from build123d import *

# Parameters (mm, degrees)
SKETCH1_R           = 3.25
BOSS_EXTRUDE1_DEPTH = 8
BOSS_EXTRUDE2_DEPTH = 12.5
BOSS_EXTRUDE3_START = -12.5
BOSS_EXTRUDE3_DEPTH = 8
SKETCH2_R           = 7.5
BOSS_EXTRUDE4_DEPTH = 10
FILLET2_R           = 2
FILLET3_R           = 5


with BuildPart() as part:
    # Sketch1 → Boss-Extrude1 (new body)
    with BuildSketch(Plane(origin=(0, 0, 0), x_dir=(1, 0, 0), z_dir=(0, 1, 0))):
        with BuildLine():
            Line((-20, 10), (-20, -10))
            Line((-20, -10), (-11.180339887, -10))
            ThreePointArc((-11.180339887, -10), (0, -15), (11.180339887, -10))
            Line((11.180339887, -10), (20, -10))
            Line((20, -10), (20, 10))
            Line((20, 10), (11.180339887, 10))
            ThreePointArc((11.180339887, 10), (0, 15), (-11.180339887, 10))
            Line((-11.180339887, 10), (-20, 10))
        make_face()
        with Locations(Location((0, 0, 0), (0, 0, 270))):
            Circle(SKETCH1_R, mode=Mode.SUBTRACT)
    extrude(amount=BOSS_EXTRUDE1_DEPTH)

    # Sketch1<3> → Boss-Extrude2 (add)
    with BuildSketch(Plane(origin=(0, 0, 0), x_dir=(1, 0, 0), z_dir=(0, 1, 0))):
        Polygon((-15, 10), (-20, 10), (-20, -10), (-15, -10), (-15, 0), align=None)
        Polygon((20, 10), (15, 10), (15, 0), (15, -10), (20, -10), align=None)
    extrude(amount=-BOSS_EXTRUDE2_DEPTH)

    # Sketch1<4> → Boss-Extrude3 (add)
    with BuildSketch(Plane(origin=(0, 0, 0), x_dir=(1, 0, 0), z_dir=(0, 1, 0)).offset(BOSS_EXTRUDE3_START)):
        with BuildLine():
            Line((-20, 10), (-20, -10))
            Line((-20, -10), (-11.180339887, -10))
            ThreePointArc((-11.180339887, -10), (0, -15), (11.180339887, -10))
            Line((11.180339887, -10), (20, -10))
            Line((20, -10), (20, 10))
            Line((20, 10), (11.180339887, 10))
            ThreePointArc((11.180339887, 10), (0, 15), (-11.180339887, 10))
            Line((-11.180339887, 10), (-20, 10))
        make_face()
    extrude(amount=-BOSS_EXTRUDE3_DEPTH)

    # Sketch2 → Boss-Extrude4 (add)
    with BuildSketch(Plane.XZ.offset(20.5)):
        with Locations(Location((0, 0, 0), (0, 0, 270))):
            Circle(SKETCH2_R)
    extrude(amount=BOSS_EXTRUDE4_DEPTH)

    # Sketch3 → Revolve1 (revolve)
    with BuildSketch(Plane.XY):
        with BuildLine():
            ThreePointArc((0, -28.863068172), (-3.8382791, -29.277061987), (-7.5, -30.5))
            Line((-7.5, -30.5), (0, -30.5))
            Line((0, -30.5), (0, -28.863068172))
        make_face()
        with BuildLine():
            Line((0, -30.5), (-7.5, -30.5))
            ThreePointArc((-7.5, -30.5), (-17.586006185, -50.701347272), (0, -64.863068172))
            Line((0, -64.863068172), (0, -30.5))
        make_face()
    revolve(axis=Axis((0, -64.863068172, 0), (0, 1, 0)))

    # Fillet2
    fillet2_edges = [part.edges().sort_by_distance(p)[0] for p in [
        (-20, -6.25, -10),
        (-20, -6.25, 10),
        (15.590169944, -20.5, 10),
        (0, -20.5, -15),
        (0, -20.5, 15),
        (-15.590169944, -20.5, -10),
        (15.590169944, -20.5, -10),
        (20, -20.5, 0),
        (-20, -20.5, 0),
        (20, -6.25, -10),
        (-15.590169944, -20.5, 10),
        (20, -6.25, 10),
    ]]
    fillet(fillet2_edges, radius=FILLET2_R)

    # Fillet3
    fillet3_edges = [part.edges().sort_by_distance(p)[0] for p in [
        (0, -20.5, 7.5),
        (-5.303300859, -30.5, -5.303300859),
    ]]
    fillet(fillet3_edges, radius=FILLET3_R)


solid = part.part
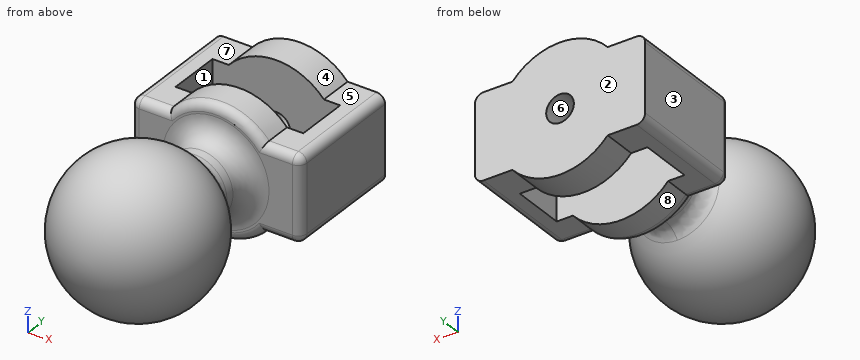
Design review of the part built by this model. Coordinates are the model's own, in mm. Face numbers are marked on the shaded views. A direction names the side the tool comes from. Give positions to 0.01 mm unless a question says otherwise; leave off trailing zeros. Order: outer loops, then holes, each group sorted by start corner. A loop starts at its lowest first (then second) coordinate and runs counter-clockwise, first axis right, second up. Notation, with made-up numbers: (71, -30) - (127, -30) arc R18 ccw to (127, -13) - close; hole circle Ø9 at (55.5, 87.5). An arc over 180 degrees is marked (long way). Use CSV: the item, a comma, the result in double quotes. Start each with the question number.
Q1. Take a section at C-C (x = -2). Count the separate pieces of the cut face and the enclosed holes in it, and give its area (3 significant figures).
Q2. Take a section at A-A (y = -6.5). State the section outline as (x, z) points, and give its area (3 significant figures).
Q3. Machinability: for the marked faces 4, 5, 6, 7 and 8, which of the approach directions +Z, -Z, +X, -X, +Y, -Y give a long, thin tool a straight path to every point of the face, cutting with its end or side? Answer none if there is none.
Q4. Draft analysis for pull direction Y (two halves, no side actions). For the marked faces 1, 2 and 3, state which applies: pulls with the +Y half, pulls with the -Y half, needs draft (parallel to the pull), parting line crosses it, or undercut.
Q5. For line 1 (Y direction, x = -6.5, z = -4.5); line 2 (X direction, y = 2.5, z = 0); line 3 (Y direction, x = 9, z = 3.5), list the stretches that pass through material, from the lowest coordinate up.
Q6. For P1, Ø3, axis at y = -57, z = -1.5, coming from the -X side; P2, Ø7.5, axis at x = 15, y = -2.5, coming from the -Z side; P3, Ø4, axis at y = -40.5, z = -9.5, coming from the +X side, all flat-tipped, find the tip position at first contact; note any pin that passes through.
Q7. Take a section at B-B (x = -16). State the section outline as (y, z) points.
Calculated:
1,separate pieces,"3"
1,enclosed holes,"0"
1,area,"1,580 mm²"
2,outline,"(-20, -8) arc R2 ccw to (-18, -10) - (-15, -10) - (-15, 10) - (-18, 10) arc R2 ccw to (-20, 8) - close; (15, -10) - (18, -10) arc R2 ccw to (20, -8) - (20, 8) arc R2 ccw to (18, 10) - (15, 10) - close"
2,area,"197 mm²"
3,face 4,"+Z, +Y"
3,face 5,"+Z, +X, +Y"
3,face 6,"+Y"
3,face 7,"+Z, -X, +Y"
3,face 8,"-Z, +Y"
4,face 1,"undercut"
4,face 2,"pulls with the +Y half"
4,face 3,"needs draft"
5,line 1,"y = -63.03 to -29.53, -23.53 to -12.5, 0 to 8"
5,line 2,"x = -20 to -3.25, 3.25 to 20"
5,line 3,"y = -62.05 to -31.67, -21.39 to -12.5, 0 to 8"
6,P1,"stops at x = -15.73"
6,P2,"stops at z = -10"
6,P3,"stops at x = 15.33"
7,outline,"circle Ø16.49 at (-46.86, 0); (-20.5, -8) arc R2 ccw to (-18.5, -10) - (8, -10) - (8, 10) - (-18.5, 10) arc R2 ccw to (-20.5, 8) - close"
